Model file for the job. Use its own axes, mm. Face numbers are marked on the shaded views. A direction names the side the tool comes from. Give positions to 0.01 mm unless a question says otherwise; leave off trailing zeros. Write each loop counter-clockwise with the first axis right and the second up, starting at its lowest first coordinate (ties: lowest second). Pieces come first, ordered by that corner, then holes. Notation, with made-up numbers: (80, -8.5) - (129, -8.5) arc R29 cw to (129, 11.5) - close; hole circle Ø8 at (73, 7.5). An arc over 180 degrees is marked (long way). One line per item, written item: value. Start each with the question number.
(1) Probe L1, parallel to Z at x = 0, y = -26.7; L2, parallel to Z at x = -3, y = -20.25; L3, parallel to Z at x = 0, y = -17.75. List the from-to ranges inside material, lowest first.
(2) Drop a flat-ended pin along its axis: P1, Ø3, axis at x = 0.5, z = 19, coming from the -Y side. Give the stop position or say it passes through.
(3) Cut at C-C, the plane y = -26.5. List the corners of the cut face in (x, z), and give its area (3 significant figures).
(4) 3-axis set-ups, long thin cutter, end or side, ignore diameter. For the marked faces 1 and 2: which of +Z, -Z, +X, -X, +Y, -Y reach the whole face in a straight line?
(5) Cut at D-D, the plane y = -19.5. State how many separate pieces and enclosed holes the cut face has, and give its area (3 significant figures).
(6) Cut at B-B, the plane x = 0. List the corners of the cut face in (y, z).
(7) Cut at A-A, the plane z = 18. List the corners of the cut face in (x, y).
(8) Mould opens along X. For the marked faces 3, 4 and 5 say: pulls with the +X half, pulls with the -X half, needs draft (parallel to the pull), parting line crosses it, or undercut.
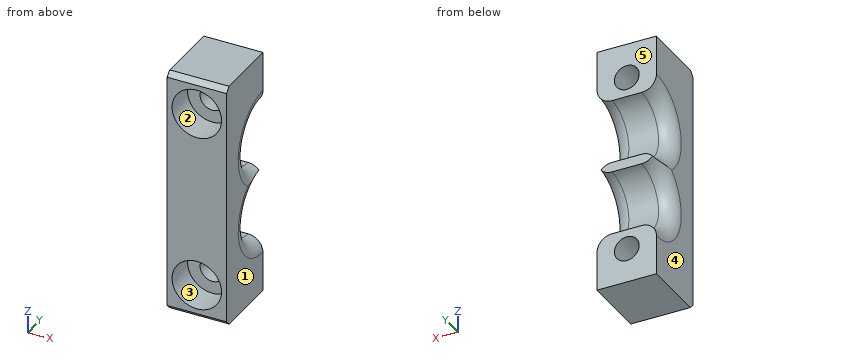
from build123d import *

# Parameters (mm, degrees)
F0_W      = 12
F0_H      = 50
F1_DEPTH  = 30
F2_R      = 6.5
F3_DEPTH  = 12.001
F4_W      = 20
F4_H      = 50
F5_DEPTH  = 2
F8_D      = 5
F9_W      = 10
F9_H      = 20
F10_DEPTH = 8
F11_R     = 5
F12_DEPTH = 6
F13_SIZE  = 1
F15_W     = 41.8421067297
F15_H     = 67.5000026822
F16_DEPTH = 25


# Not quite as in the source:
# - a fillet or chamfer that OpenCascade refuses, or shapes differently, is made with other operations: its cross-section is extruded or revolved along the edge and cut away or added


with BuildPart() as f1:
    # F0 (on Front) → F1 (new body)
    with BuildSketch(Plane.XZ):
        Rectangle(F0_W, F0_H)
    extrude(amount=F1_DEPTH)

    # F2 (on face) → F3 (cut, through all)
    with BuildSketch(Plane.YZ.offset(6)):
        with Locations((-16, 7.5)):
            Circle(F2_R)
        with Locations((-16, -7.5)):
            Circle(F2_R)
    extrude(amount=-F3_DEPTH, mode=Mode.SUBTRACT)

    # F4 (on Front) → F5 (join)
    with BuildSketch(Plane.XZ):
        Rectangle(F4_W, F4_H)
    extrude(amount=F5_DEPTH)

    # F6: fillet of radius 3 on 4 edges, made by hand

    # F6_s1 → F6_t2 (revolve, cut)
    with BuildSketch(Plane.XY.offset(7.5)):
        with BuildLine():
            ThreePointArc((-6, -6.5), (-5.1213203436, -8.6213203436), (-3, -9.5))
            Line((-3, -9.5), (-6, -9.5))
            Line((-6, -9.5), (-6, -6.5))
        make_face()
    revolve(axis=Axis((-6, -16, 7.5), (1, 0, 0)), mode=Mode.SUBTRACT)

    # F6_s3 → F6_t4 (revolve, cut)
    with BuildSketch(Plane.XY.offset(-7.5)):
        with BuildLine():
            ThreePointArc((-6, -6.5), (-5.1213203436, -8.6213203436), (-3, -9.5))
            Line((-3, -9.5), (-6, -9.5))
            Line((-6, -9.5), (-6, -6.5))
        make_face()
    revolve(axis=Axis((-6, -16, -7.5), (1, 0, 0)), mode=Mode.SUBTRACT)

    # F6_s5 → F6_t6 (revolve, cut)
    with BuildSketch(Plane.XY.offset(7.5)):
        with BuildLine():
            ThreePointArc((3, -9.5), (5.1213203436, -8.6213203436), (6, -6.5))
            Line((6, -6.5), (6, -9.5))
            Line((6, -9.5), (3, -9.5))
        make_face()
    revolve(axis=Axis((6, -16, 7.5), (1, 0, 0)), mode=Mode.SUBTRACT)

    # F6_s7 → F6_t8 (revolve, cut)
    with BuildSketch(Plane.XY.offset(-7.5)):
        with BuildLine():
            ThreePointArc((3, -9.5), (5.1213203436, -8.6213203436), (6, -6.5))
            Line((6, -6.5), (6, -9.5))
            Line((6, -9.5), (3, -9.5))
        make_face()
    revolve(axis=Axis((6, -16, -7.5), (1, 0, 0)), mode=Mode.SUBTRACT)

    # F8 (through all)
    with Locations(Plane(origin=(0, 0, 0), x_dir=(-1, 0, 0), z_dir=(0, 1, 0))):
        with Locations((0, 18), (0, -18)):
            Hole(F8_D / 2)

    # F9 (on face) → F10 (cut)
    with BuildSketch(Plane(origin=(0, 0, 0), x_dir=(-1, 0, 0), z_dir=(0, 1, 0))):
        Polygon((0, 12.1110272543), (5.1, 15.0555136271), (5.1, 20.9444863729), (0, 23.8889727457), (-5.1, 20.9444863729), (-5.1, 15.0555136271), align=None)
        Rectangle(F9_W, F9_H)
        Polygon((5.1, -20.9444863729), (5.1, -15.0555136271), (0, -12.1110272543), (-5.1, -15.0555136271), (-5.1, -20.9444863729), (0, -23.8889727457), align=None)
    extrude(amount=-F10_DEPTH, mode=Mode.SUBTRACT)

    # F11 (on face) → F12 (cut)
    with BuildSketch(Plane.XZ.offset(30)):
        with Locations((0, 18)):
            Circle(F11_R)
        with Locations((0, -18)):
            Circle(F11_R)
    extrude(amount=-F12_DEPTH, mode=Mode.SUBTRACT)

    # F13
    f13_edges = [f1.edges().sort_by_distance(p)[0] for p in [
        (0, -30, -25),
        (0, -30, 25),
    ]]
    chamfer(f13_edges, length=F13_SIZE)

    # F15 (on offset) → F16 (cut)
    with BuildSketch(Plane.XZ.offset(16)):
        with Locations((-0.493420288, -0.09868294)):
            Rectangle(F15_W, F15_H)
    extrude(amount=-F16_DEPTH, mode=Mode.SUBTRACT)


solid = f1.part
Answers follow:
1. L1: z = -25 to -23, -13 to 13, 23 to 25
1. L2: z = -25 to -12.42, -2.58 to 2.58, 12.42 to 25
1. L3: z = -25 to -20.5, -15.5 to -13.76, -1.24 to 1.24, 13.76 to 15.5, 20.5 to 25
2. P1: stops at y = -24
3. outline: (-6, -25) - (6, -25) - (6, 25) - (-6, 25) - close; hole circle Ø10 at (0, -18); hole circle Ø10 at (0, 18)
3. area: 443 mm²
4. face 1: +Z, -Z, +X, +Y, -Y
4. face 2: -Y
5. separate pieces: 3
5. enclosed holes: 2
5. area: 281 mm²
6. outline: (-30, -24) - (-29, -25) - (-16, -25) - (-16, -20.5) - (-24, -20.5) - (-24, -23) - (-30, -23) - close; (-30, -13) - (-24, -13) - (-24, -15.5) - (-16, -15.5) - (-16, -14) arc R6.5 cw to (-16, -1) - (-16, 1) arc R6.5 cw to (-16, 14) - (-16, 15.5) - (-24, 15.5) - (-24, 13) - (-30, 13) - close; (-30, 23) - (-24, 23) - (-24, 20.5) - (-16, 20.5) - (-16, 25) - (-29, 25) - (-30, 24) - close
7. outline: (-6, -30) - (-5, -30) - (-5, -24) - (-2.5, -24) - (-2.5, -16) - (-6, -16) - close; (2.5, -24) - (5, -24) - (5, -30) - (6, -30) - (6, -16) - (2.5, -16) - close
8. face 3: undercut
8. face 4: pulls with the -X half
8. face 5: needs draft
